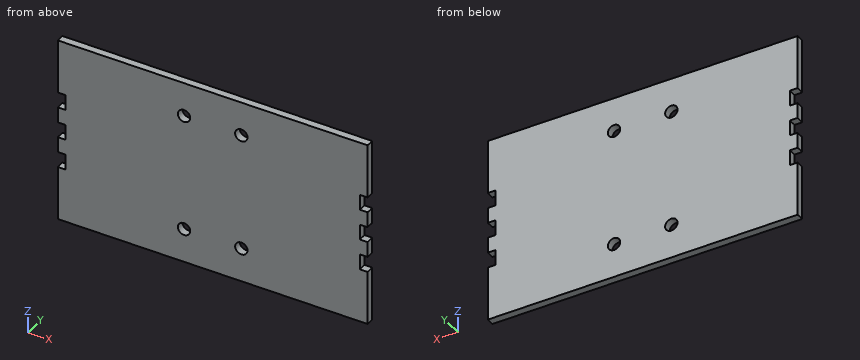
from build123d import *

# Parameters (mm, degrees)
SKETCH_1_W          = 200
SKETCH_1_H          = 120
EXTRUDE_1_DEPTH     = 5
SKETCH_2_W          = 5
SKETCH_2_H          = 10
CUT_EXTRUDE_1_DEPTH = 5
SKETCH_3_R          = 4
CUT_EXTRUDE_2_DEPTH = 6


with BuildPart() as part:
    # 草图1 → 凸台-拉伸1 (new body)
    with BuildSketch(Plane(origin=(0, 0, 0), x_dir=(1, 0, 0), z_dir=(0, 1, 0))):
        Rectangle(SKETCH_1_W, SKETCH_1_H)
    extrude(amount=EXTRUDE_1_DEPTH)

    # 草图2 → 切除-拉伸1 (cut)
    with BuildSketch(Plane(origin=(0, 5, 0), x_dir=(1, 0, 0), z_dir=(0, 1, 0))):
        with Locations((97.5, 0)):
            Rectangle(SKETCH_2_W, SKETCH_2_H)
        with Locations((-97.5, 0)):
            Rectangle(SKETCH_2_W, SKETCH_2_H)
        with Locations((-97.5, -20)):
            Rectangle(SKETCH_2_W, SKETCH_2_H)
        with Locations((-97.5, 20)):
            Rectangle(SKETCH_2_W, SKETCH_2_H)
        with Locations((97.5, -20)):
            Rectangle(SKETCH_2_W, SKETCH_2_H)
        with Locations((97.5, 20)):
            Rectangle(SKETCH_2_W, SKETCH_2_H)
    extrude(amount=-CUT_EXTRUDE_1_DEPTH, mode=Mode.SUBTRACT)

    # 草图3 → 切除-拉伸2 (cut, through all)
    with BuildSketch(Plane(origin=(0, 5, 0), x_dir=(1, 0, 0), z_dir=(0, 1, 0))):
        with Locations((-18.5, 38)):
            Circle(SKETCH_3_R)
        with Locations((18.5, 38)):
            Circle(SKETCH_3_R)
        with Locations((18.5, -38)):
            Circle(SKETCH_3_R)
        with Locations((-18.5, -38)):
            Circle(SKETCH_3_R)
    extrude(amount=-CUT_EXTRUDE_2_DEPTH, mode=Mode.SUBTRACT)


solid = part.part
Read the model definition and answer for the solid it produces. Units are mm, in the model's axes. Coordinates: 2 decimals unless noted, no trailing zeros. Order: outer loops, then holes, each group sorted by start corner. A loop starts at its lowest first (then second) coordinate and runs counter-clockwise, first axis right, second up. Notation, with made-up numbers: (-25, 30.5) -> (-6, 30.5) arc R25 cw to (-6, 49.5) -> close; hole circle Ø3 at (-23, 32). An arc over 180 degrees is marked (long way). Answer as a JSON object with one key per item and string values.
1) Each of these flat-tipped pins is pushed along its axis until it touches: pin 1 (1.5 mm diameter, centred on y = 2, z = 21.5, fed in from +X); pin 2 (2.5 mm diameter, centred on y = 2, z = -0.5, fed in from -X). Where does it stop, or does it pass through?
Model answer:
{"pin 1": "stops at x = 95", "pin 2": "stops at x = -95"}
2) A cutting plane is placed at C-C, the plane y = 3.15. State how many separate pieces and enclosed holes the cut face has, plus the area to 3 significant figures.
Model answer:
{"separate pieces": "1", "enclosed holes": "4", "area": "23,500 mm²"}
3) A cutting plane is placed at B-B, the plane x = -18.5. Determine the outline of the cut face in (y, z).
Model answer:
{"outline": "(0, -60) -> (5, -60) -> (5, -42) -> (0, -42) -> close; (0, -34) -> (5, -34) -> (5, 34) -> (0, 34) -> close; (0, 42) -> (5, 42) -> (5, 60) -> (0, 60) -> close"}
4) A cutting plane is placed at A-A, the plane z = 38. Determine the outline of the cut face in (x, y).
Model answer:
{"outline": "(-100, 0) -> (-22.5, 0) -> (-22.5, 5) -> (-100, 5) -> close; (-14.5, 0) -> (14.5, 0) -> (14.5, 5) -> (-14.5, 5) -> close; (22.5, 0) -> (100, 0) -> (100, 5) -> (22.5, 5) -> close"}
5) A cutting plane is placed at D-D, the plane z = -0.5. Determine the outline of the cut face in (x, y).
Model answer:
{"outline": "(-95, 0) -> (95, 0) -> (95, 5) -> (-95, 5) -> close"}
6) Consider line 1 along X through (y, z) = (1.4, -38); line 2 along Z through (x, y) = (-18.5, 3.15); line 3 along X through (y, z) = (3.05, -35). Determine where each line is inside the solid, lowest interval first. Write a range as from..to.
Model answer:
{"line 1": "x = -100..-22.5, -14.5..14.5, 22.5..100", "line 2": "z = -60..-42, -34..34, 42..60", "line 3": "x = -100..-21.15, -15.85..15.85, 21.15..100"}
